Design review of the part built by this model. Coordinates are the model's own, in mm. Face numbers are marked on the shaded views. Round coordinates to 2 decimals unless told otherwise and drop trailing zeros. Order: outer loops, then holes, each group sorted by start corner. A loop starts at its lowest first (then second) coordinate and runs counter-clockwise, first axis right, second up. Notation, with made-up numbers: M -17,71.5 L -2,71.5 A20 cw -2,83.5 Z; hole C 71.5,89.5 d4. An arc over 180 degrees is marked long. Use a Markdown table: item, result. Add a question column.
(1) For pin 1 (2 mm diameter, centred on x = -15, y = 12.5, fed in from +Z); pin 2 (10 mm diameter, centred on y = 39.5, z = -34.5, fed in from -X), all flat-tipped, find the tip position at first contact; note any pin that passes through.
(2) Take a section at C-C (y = 53). Write out the cut boundary in (x, z), then the cut area to 3 significant figures.
(3) The part is to be moulded in two halves that separate along Y. For the marked faces 1, 2 and 3, say which applies: released by +Y, released by -Y, zero draft, split by the parting line, or undercut.
(4) Take a section at A-A (x = 0). Write out the cut boundary in (y, z).
(5) Take a section at D-D (z = 61). Write out the cut boundary in (x, y), then the cut area to 3 significant figures.
(6) To check wall thickness, follow probe 1 along Z at (x, y) = (0, 70.75); probe 2 along Y at (x, z) = (-5, 34); probe 3 along X at (y, z) = (41, -50). State the ranges of each line that lie inside material, in increasing order. Write a range as from..to.
(7) Take a section at B-B (z = 7). Write out the cut boundary in (x, y), then the cut area to 3 significant figures.
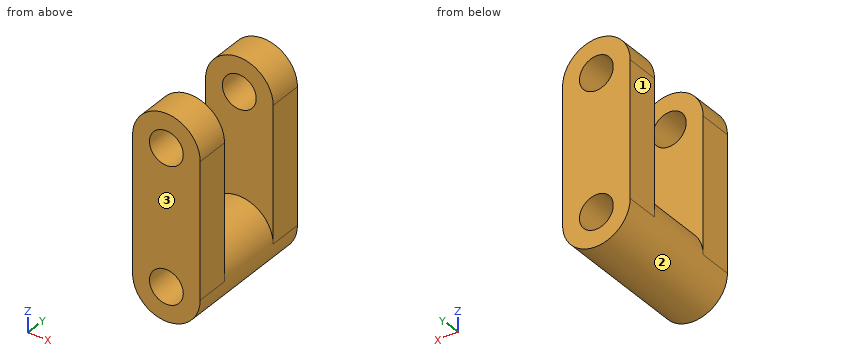
```python
from build123d import *

# Parameters (mm, degrees)
F0_R     = 12.7
F1_DEPTH = 25.4
F2_R     = 25.4
F3_DEPTH = 25.4
F4_R     = 12.7
F5_DEPTH = 50.801


with BuildPart() as f1:
    # F0 (on Front) → F1 (new body)
    with BuildSketch(Plane.XZ):
        with BuildLine():
            ThreePointArc((25.4, 50.8), (0, 76.2), (-25.4, 50.8))
            Line((-25.4, 50.8), (-25.4, -50.8))
            ThreePointArc((-25.4, -50.8), (0, -76.2), (25.4, -50.8))
            Line((25.4, -50.8), (25.4, 50.8))
        make_face()
        with Locations((0, -50.8)):
            Circle(F0_R, mode=Mode.SUBTRACT)
        with Locations((0, 50.8)):
            Circle(F0_R, mode=Mode.SUBTRACT)
    extrude(amount=F1_DEPTH)

    # F2 (on face) → F3 (join)
    with BuildSketch(Plane(origin=(0, 0, 0), x_dir=(-1, 0, 0), z_dir=(0, 1, 0))):
        with Locations((0, -50.8)):
            Circle(F2_R)
    extrude(amount=F3_DEPTH)

    # F4 (on face) → F5 (cut, through all)
    with BuildSketch(Plane.XZ.offset(25.4)):
        with Locations((0, -50.8)):
            Circle(F4_R)
    extrude(amount=-F5_DEPTH, mode=Mode.SUBTRACT)

    # F6: F1 across face


with BuildPart() as f1_1:
    add(f1.part)
    add(f1.part.mirror(Plane(origin=(0, 25.4, -50.8), x_dir=(-1, 0, 0), z_dir=(0, 1, 0))))


solid = f1_1.part
```
Verdict:
| question | item | result |
|---|---|---|
| 1 | pin 1 | stops at z = -29.61 |
| 1 | pin 2 | stops at x = -22.75 |
| 2 | outline | M -25.4,-50.8 A25.4 ccw 25.4,-50.8 L 25.4,50.8 A25.4 ccw -25.4,50.8 Z; hole C 0,-50.8 d25.4; hole C 0,50.8 d25.4 |
| 2 | area | 6,170 mm^2 |
| 3 | face 1 | zero draft |
| 3 | face 2 | undercut |
| 3 | face 3 | released by -Y |
| 4 | outline | M -25.4,-76.2 L 76.2,-76.2 L 76.2,-63.5 L -25.4,-63.5 Z; M -25.4,-38.1 L 76.2,-38.1 L 76.2,38.1 L 50.8,38.1 L 50.8,-25.4 L 0,-25.4 L 0,38.1 L -25.4,38.1 Z; M -25.4,63.5 L 0,63.5 L 0,76.2 L -25.4,76.2 Z; M 50.8,63.5 L 76.2,63.5 L 76.2,76.2 L 50.8,76.2 Z |
| 5 | outline | M -23.26,-25.4 L -7.57,-25.4 L -7.57,0 L -23.26,0 Z; M -23.26,50.8 L -7.57,50.8 L -7.57,76.2 L -23.26,76.2 Z; M 7.57,-25.4 L 23.26,-25.4 L 23.26,0 L 7.57,0 Z; M 7.57,50.8 L 23.26,50.8 L 23.26,76.2 L 7.57,76.2 Z |
| 5 | area | 1,590 mm^2 |
| 6 | probe 1 | z = -76.2..-63.5, -38.1..38.1, 63.5..76.2 |
| 6 | probe 2 | y = -25.4..0, 50.8..76.2 |
| 6 | probe 3 | x = -25.39..-12.67, 12.67..25.39 |
| 7 | outline | M -25.4,-25.4 L 25.4,-25.4 L 25.4,0 L -25.4,0 Z; M -25.4,50.8 L 25.4,50.8 L 25.4,76.2 L -25.4,76.2 Z |
| 7 | area | 2,580 mm^2 |
